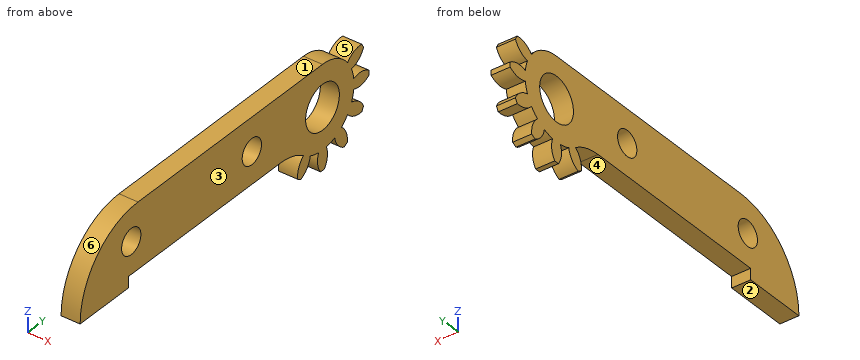
```python
from build123d import *

# Parameters (mm, degrees)
CROQUIS1_R              = 2
CROQUIS1_R_2            = 3.5
SALIENTE_EXTRUIR1_DEPTH = 3


with BuildPart() as part:
    # Croquis1 → Saliente-Extruir1 (new body)
    with BuildSketch(Plane(origin=(2.816112381, 0, 0), x_dir=(0, 0, -1), z_dir=(1, 0, 0))):
        with BuildLine():
            Line((-6.304052244, 0.230126664), (-6.304052244, -38))
            ThreePointArc((-6.304052244, -38), (-2.789333619, -46.485281374), (5.695947756, -50))
            Line((5.695947756, -50), (5.695947756, -40))
            Line((5.695947756, -40), (3.945947756, -40))
            Line((3.945947756, -40), (3.945947756, -8.356393503))
            ThreePointArc((3.945947756, -8.356393503), (4.325796585, -5.920557684), (5.42927179, -3.716034211))
            ThreePointArc((5.42927179, -3.716034211), (6.741018488, -4.690759176), (8.359590341, -4.916576169))
            ThreePointArc((8.359590341, -4.916576169), (8.561692267, -4.582373336), (8.750069448, -4.240246517))
            ThreePointArc((8.750069448, -4.240246517), (7.745220269, -2.951430671), (6.245210338, -2.302787189))
            ThreePointArc((6.245210338, -2.302787189), (6.533934883, -1.460026405), (6.705272485, -0.585811884))
            ThreePointArc((6.705272485, -0.585811884), (8.328640931, -0.774075116), (9.84327377, -0.160352443))
            ThreePointArc((9.84327377, -0.160352443), (9.851197756, 0.230126664), (9.84327377, 0.620605771))
            ThreePointArc((9.84327377, 0.620605771), (8.328640931, 1.234328445), (6.705272485, 1.046065213))
            ThreePointArc((6.705272485, 1.046065213), (6.533934883, 1.920279734), (6.245210338, 2.763040518))
            ThreePointArc((6.245210338, 2.763040518), (7.745220269, 3.411683999), (8.750069448, 4.700499845))
            ThreePointArc((8.750069448, 4.700499845), (8.561692267, 5.042626664), (8.359590341, 5.376829498))
            ThreePointArc((8.359590341, 5.376829498), (6.741018488, 5.151012505), (5.42927179, 4.17628754))
            ThreePointArc((5.42927179, 4.17628754), (4.843781813, 4.847710722), (4.172358631, 5.433200699))
            ThreePointArc((4.172358631, 5.433200699), (5.147083596, 6.744947397), (5.372900589, 8.363519249))
            ThreePointArc((5.372900589, 8.363519249), (5.038697756, 8.565621176), (4.696570936, 8.753998356))
            ThreePointArc((4.696570936, 8.753998356), (3.407755091, 7.749149177), (2.759111609, 6.249139247))
            ThreePointArc((2.759111609, 6.249139247), (1.916350825, 6.537863791), (1.042136304, 6.709201394))
            ThreePointArc((1.042136304, 6.709201394), (1.230399536, 8.33256984), (0.616676863, 9.847202679))
            ThreePointArc((0.616676863, 9.847202679), (0.226197756, 9.855126664), (-0.164281352, 9.847202679))
            ThreePointArc((-0.164281352, 9.847202679), (-0.778004025, 8.33256984), (-0.589740793, 6.709201394))
            ThreePointArc((-0.589740793, 6.709201394), (-1.463955314, 6.537863791), (-2.306716098, 6.249139247))
            ThreePointArc((-2.306716098, 6.249139247), (-2.95535958, 7.749149177), (-4.244175425, 8.753998356))
            ThreePointArc((-4.244175425, 8.753998356), (-4.586302244, 8.565621176), (-4.920505078, 8.363519249))
            ThreePointArc((-4.920505078, 8.363519249), (-4.694688085, 6.744947397), (-3.71996312, 5.433200699))
            ThreePointArc((-3.71996312, 5.433200699), (-5.622459446, 3.134842486), (-6.304052244, 0.230126664))
        make_face()
        with Locations((-1.054052244, -14.410797367)):
            Circle(CROQUIS1_R, mode=Mode.SUBTRACT)
        with Locations((-1.054052244, -39.410797367)):
            Circle(CROQUIS1_R, mode=Mode.SUBTRACT)
        with Locations((0.226197756, 0.230126664)):
            Circle(CROQUIS1_R_2, mode=Mode.SUBTRACT)
    extrude(amount=-SALIENTE_EXTRUIR1_DEPTH)


solid = part.part
```
Geometry check sheet. Reference: the model listing, model coordinates, mm. Face numbers are marked on the shaded views. A direction names the side the tool comes from. Coordinates: 2 decimals unless noted, no trailing zeros. Loops run counter-clockwise (first coordinate to the right, second up) from the corner with the lowest first, then second, coordinate; pieces in that order, holes last.
Item 1: Sectioned sample at A-A, the plane z = -2.25. Record the boundary of the cut face in (x, y), then the cut area to 3 significant figures.
Item 2: Sectioned sample at B-B, the plane x = 2.3. Count the separate pieces of the cut face and the enclosed holes in it, then the cut area to 3 significant figures.
Item 3: Go/stop test with flat-tipped pins: pin 1 Ø1.4 at (x, z) = (1.5, -5) entering from +Y; pin 2 Ø3 at (y, z) = (-39.41, 1.05) entering from +X; pin 3 Ø1.5 at (x, y) = (0.5, -46.5) entering from -Z; pin 4 Ø1.5 at (x, y) = (0.5, -30) entering from -Z. Record where each tip stops, or that it passes through.
Item 4: Thickness scan on line 1 (Z direction, x = 1.8, y = 0.5); line 2 (Y direction, x = 1.9, z = -7.5); line 3 (Y direction, x = 1.8, z = 1.5). Record the ranges inside material, lowest first.
Item 5: Release check for a two-part mould opening along Y. For the marked faces 3, 4, 5 and 6 record: released by +Y, released by -Y, zero draft, split by the parting line, or undercut.
Item 6: Access from +Z, -Z, +X, -X, +Y, -Y to the whole of each face (thin tool, end or side, straight path). Record for the marked faces 1 and 2.
Item 7: Sectioned sample at C-C, the plane y = -33. Record the boundary of the cut face in (x, z).
Item 8: Sectioned sample at D-D, the plane y = -46. Record the boundary of the cut face in (x, z), then the cut area to 3 significant figures.
Check result:
1. outline: (-0.18, -49.49) - (2.82, -49.49) - (2.82, -2.63) - (-0.18, -2.63) - close; (-0.18, 3.09) - (2.82, 3.09) - (2.82, 6.44) - (-0.18, 6.44) - close
1. area: 151 mm2
2. separate pieces: 1
2. enclosed holes: 3
2. area: 549 mm2
3. pin 1: stops at y = 8.75
3. pin 2: passes through
3. pin 3: stops at z = -5.7
3. pin 4: stops at z = -3.95
4. line 1: z = -9.85 to -3.72, 3.26 to 6.3
4. line 2: y = -4.9 to -2.78, -0.78 to 1.24, 3.24 to 5.36
4. line 3: y = -47.6 to -41.36, -37.46 to -16.36, -12.46 to -2.81, 3.27 to 6.53
5. face 3: zero draft
5. face 4: undercut
5. face 5: undercut
5. face 6: released by -Y
6. face 1: +Z, +X, -X, +Y, -Y
6. face 2: -Z, +X, -X, -Y
7. outline: (-0.18, -3.95) - (2.82, -3.95) - (2.82, 6.3) - (-0.18, 6.3) - close
8. outline: (-0.18, -5.7) - (2.82, -5.7) - (2.82, 3.25) - (-0.18, 3.25) - close
8. area: 26.8 mm2
